from build123d import *

# Parameters (mm, degrees)
SKETCH1_W           = 41.185763127
SKETCH1_H           = 12.7
BOSS_EXTRUDE1_DEPTH = 5.08
SKETCH3_W           = 1.801844016
SKETCH3_H           = 1.294077433
BOSS_EXTRUDE2_DEPTH = 2.54


with BuildPart() as part:
    # Sketch1 → Boss-Extrude1 (new body)
    with BuildSketch(Plane(origin=(0, 0, 0), x_dir=(1, 0, 0), z_dir=(0, 1, 0))):
        with Locations((17.507118437, 6.35)):
            Rectangle(SKETCH1_W, SKETCH1_H)
        with BuildLine():
            ThreePointArc((28.547464109, 6.35), (31.722464109, 9.968769047), (34.897464109, 6.35))
            ThreePointArc((34.897464109, 6.35), (31.722464109, 3.175), (28.547464109, 6.35))
        make_face(mode=Mode.SUBTRACT)
        with BuildLine():
            ThreePointArc((14.915366262, 6.35), (19.677866262, 11.860840795), (24.440366262, 6.35))
            ThreePointArc((24.440366262, 6.35), (19.677866262, 1.5875), (14.915366262, 6.35))
        make_face(mode=Mode.SUBTRACT)
        with BuildLine():
            ThreePointArc((0.879836225, 6.35), (5.379836225, 11.549994731), (9.879836225, 6.35))
            ThreePointArc((9.879836225, 6.35), (5.379836225, 1.85), (0.879836225, 6.35))
        make_face(mode=Mode.SUBTRACT)
    extrude(amount=BOSS_EXTRUDE1_DEPTH)

    # Sketch3 → Boss-Extrude2 (add)
    with BuildSketch(Plane(origin=(0, 5.08, 0), x_dir=(1, 0, 0), z_dir=(0, 1, 0))):
        with Locations((-2.184841119, 0.647038716)):
            Rectangle(SKETCH3_W, SKETCH3_H)
    extrude(amount=BOSS_EXTRUDE2_DEPTH)


solid = part.part
The model under review builds one solid part; all positions refer to its coordinate system, in mm. A direction names the side the tool comes from. Give positions to 0.01 mm unless a question says otherwise; leave off trailing zeros. Loops run counter-clockwise (first coordinate to the right, second up) from the corner with the lowest first, then second, coordinate; pieces in that order, holes last. Notation, with made-up numbers: (28.25, -38.75) -> (81.25, -38.75) arc R22 cw to (81.25, -17.75) -> close; hole circle Ø1 at (40, 82). An arc over 180 degrees is marked (long way). Put each result on its own line as item: value. Start each with the question number.
1. We need section B-B on y = 4. State how many separate pieces and enclosed holes the cut face has, then the cut area to 3 significant figures.
2. We need section D-D on x = 23.5. State the section outline as (y, z) points.
3. For faces 1 (the face through (19.78, 2.5, -1.59)), 2 (the face through (-2, 6, -1.294)), 3 (the face through (-1.284, 6, -1)), list the 3-axis set-ups (+Z, -Z, +X, -X, +Y, -Y) from which the entire face can be reached by the end or side of a thin tool; tool diameter is ignored.
4. Mouldability with a two-part tool opening along Z and no side actions: class faces 4 (the face through (38.1, 3, -6)), 5 (the face through (17, 3, -12.7)), 6 (the face through (5.48, 2.5, -1.85)) as released by +Z, released by -Z, zero draft, split by the parting line, or undercut.
5. We need section A-A on z = -10.75. State the section outline as (x, y) points, then the cut area to 3 significant figures.
6. Clearance check with flat-ended pins moving along their axes: P1, Ø3, axis at y = 5.5, z = -11, coming from the +X side; P2, Ø4, axis at x = 13, z = -5, coming from the +Y side; P3, Ø6, axis at x = 19.68, z = -7.05, coming from the -Y side; P4, Ø1.4, axis at x = -2, y = 7, coming from the -Z side. State where each tip first meets the part, or that it passes through.
7. We need section C-C on x = 9.5. State the section outline as (y, z) points, then the cut area to 3 significant figures.
8. Wall thickness on probe 1 along X at (y, z) = (1.5, -4.75); probe 2 along Y at (x, z) = (35, -5); probe 3 along Z at (x, y) = (3.5, 4.5): over which ranges is each line inside the solid? List them lowest first.
Determined:
1. separate pieces: 1
1. enclosed holes: 3
1. area: 340 mm^2
2. outline: (0, -12.7) -> (5.08, -12.7) -> (5.08, -9.97) -> (0, -9.97) -> close; (0, -3.51) -> (5.08, -3.51) -> (5.08, 0) -> (0, 0) -> close
3. face 1: +Y, -Y
3. face 2: -Z, +X, -X, +Y
3. face 3: +Z, -Z, +X, +Y
4. face 4: zero draft
4. face 5: released by -Z
4. face 6: undercut
5. outline: (-3.09, 0) -> (2.8, 0) -> (2.8, 5.08) -> (-3.09, 5.08) -> close; (7.96, 0) -> (16.6, 0) -> (16.6, 5.08) -> (7.96, 5.08) -> close; (22.75, 0) -> (38.1, 0) -> (38.1, 5.08) -> (22.75, 5.08) -> close
5. area: 152 mm^2
6. P1: x = 38.1
6. P2: y = 5.08
6. P3: through
6. P4: z = -1.29
7. outline: (0, -12.7) -> (5.08, -12.7) -> (5.08, -8.93) -> (0, -8.93) -> close; (0, -4.54) -> (5.08, -4.54) -> (5.08, 0) -> (0, 0) -> close
7. area: 42.2 mm^2
8. probe 1: -3.09 to 1.17, 9.59 to 15.19, 24.16 to 28.98, 34.46 to 38.1
8. probe 2: 0 to 5.08
8. probe 3: -12.7 to -11.14, -2.26 to 0
